```python
from build123d import *

# Parameters (mm, degrees)
SKETCH1_R           = 10
SKETCH1_R_2         = 2
BOSS_EXTRUDE1_DEPTH = 7.5
BOSS_EXTRUDE2_START = 7
SKETCH2_R           = 10
SKETCH2_R_2         = 4.125
BOSS_EXTRUDE2_DEPTH = 7
SKETCH3_R           = 4
CUT_EXTRUDE1_DEPTH  = 3
CUT_EXTRUDE1_DRAFT  = -34
FILLET1_R           = 5
FILLET2_R           = 1


with BuildPart() as part:
    # Sketch1 → Boss-Extrude1 (new body)
    with BuildSketch(Plane(origin=(0, 0, 0), x_dir=(1, 0, 0), z_dir=(0, 1, 0))):
        with Locations(Location((0, 0, 0), (0, 0, 270))):
            Circle(SKETCH1_R)
        with Locations(Location((0, 0, 0), (0, 0, 270))):
            Circle(SKETCH1_R_2, mode=Mode.SUBTRACT)
    extrude(amount=BOSS_EXTRUDE1_DEPTH)

    # Sketch2 → Boss-Extrude2 (add)
    with BuildSketch(Plane.XZ.offset(BOSS_EXTRUDE2_START)):
        with Locations(Location((0, 0, 0), (0, 0, 270))):
            Circle(SKETCH2_R)
        with Locations(Location((0, 0, 0), (0, 0, 270))):
            Circle(SKETCH2_R_2, mode=Mode.SUBTRACT)
    extrude(amount=-BOSS_EXTRUDE2_DEPTH)


with BuildPart() as cut_extrude1_tool:
    # Sketch3 → Cut-Extrude1 (with draft: the straight prism first)
    with BuildSketch(Plane(origin=(0, 7.5, 0), x_dir=(1, 0, 0), z_dir=(0, 1, 0))):
        Circle(SKETCH3_R)
    extrude(amount=-CUT_EXTRUDE1_DEPTH)
    # Cut-Extrude1: the draft: its side faces are tilted about the plane it starts from
    cut_extrude1_sides = [cut_extrude1_tool.faces().sort_by_distance(p)[0] for p in [
        (-4, 6, 0),
    ]]
    draft(cut_extrude1_sides, Plane(origin=(0, 7.5, 0), x_dir=(1, 0, 0), z_dir=(0, 1, 0)), CUT_EXTRUDE1_DRAFT)


with BuildPart() as part_1:
    add(part.part)

    # Cut-Extrude1: cut by cut_extrude1_tool
    add(cut_extrude1_tool.part, mode=Mode.SUBTRACT)

    # Fillet1
    fillet1_edges = [part_1.edges().sort_by_distance(p)[0] for p in [
        (0, 7.5, -10),
    ]]
    fillet(fillet1_edges, radius=FILLET1_R)

    # Fillet2
    fillet2_edges = [part_1.edges().sort_by_distance(p)[0] for p in [
        (0, -7, 4.125),
    ]]
    fillet(fillet2_edges, radius=FILLET2_R)


solid = part_1.part
```
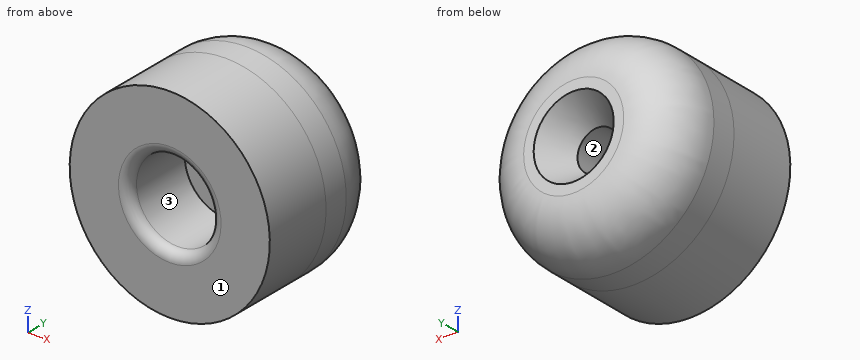
Part model, mm, in its own coordinate system. Face numbers are marked on the shaded views. Coordinates: 2 decimals unless noted, no trailing zeros. Order: outer loops, then holes, each group sorted by start corner. A loop starts at its lowest first (then second) coordinate and runs counter-clockwise, first axis right, second up. Notation, with made-up numbers: (27, 44.5) - (60, 44.5) arc R22 cw to (60, 52.5) - close; hole circle Ø7 at (4, 66). An arc over 180 degrees is marked (long way). Return JSON: item names as keys, results as strings. Group by question number.
Item 1: Cut at B-B (y = 0.75). List the corners of the cut face in (x, z), plus the area to 3 significant figures.
Item 2: Pin check, flat tips, straight feed: pin 1 (5 mm diameter, centred on x = 4, y = -5.5, fed in from -Z); pin 2 (6 mm diameter, centred on x = -4.5, z = 7, fed in from +Y); pin 3 (3 mm diameter, centred on y = 2, z = 7.5, fed in from -X). Stop position of each tip, or through.
Item 3: Drill centre lines: probe 1 along X at (y, z) = (1.2, 0); probe 2 along X at (y, z) = (-2.6, 0) (3 decimals); probe 3 along Z at (x, y) = (-0.5, 6.5). Where is each one in solid material? Low to high. Write a range as from..to.
Item 4: Cut at A-A (y = -2.5). List the corners of the cut face in (x, z) (3 decimals).
Item 5: Pull direction Z, two halves, no side cores. Call the marked faces 1, 2 and 3: pulls with the +Z half, pulls with the -Z half, needs draft (parallel to the pull), parting line crosses it, or undercut.
Check values:
{
 "1": {"outline": "circle Ø20 at (0, 0); hole circle Ø4 at (0, 0)", "area": "302 mm2"},
 "2": {"pin 1": "stops at z = -9.89", "pin 2": "stops at y = 7.49", "pin 3": "stops at x = -8"},
 "3": {"probe 1": "x = -10..-2, 2..10", "probe 2": "x = -10..-4.125, 4.125..10", "probe 3": "z = -7.98..-3.29, 3.29..7.98"},
 "4": {"outline": "circle Ø20 at (0, 0); hole circle Ø8.25 at (0, 0)"},
 "5": {"face 1": "needs draft", "face 2": "undercut", "face 3": "undercut"}
}
